Could you check a few things on this drawing? It's one solid part, dimensions in mm from its lowest x, y, z. A direction names the side the tool comes from. Give positions to 0.01 mm unless a question says otherwise; leave off trailing zeros. Write each loop counter-clockwise with the first axis right and the second up, starting at its lowest first coordinate (ties: lowest second). Pieces come first, ordered by that corner, then holes. Notation, with made-up numbers: (71, -13) -> (115, -13) arc R38 cw to (115, 26) -> close; hole circle Ø2 at (62, 39). An arc over 180 degrees is marked (long way). Use CSV: the item, a comma, the result in double quotes. Start each with the question number.
(1) I need wall thicknesses on L1, parallel to Y at x = 14, z = 4 (1 decimal); L2, parallel to Z at x = 11.75, y = 17.5 (1 decimal); L3, parallel to Y at x = 10.5, z = 8 (1 decimal). Which ranges of each line are inside material? Lowest first, please. Write a range as [from, to].
(2) Suppose I cut it at B-B on z = 4.25. List the corners of the cut face in (x, y) for me (1 decimal).
(3) Suppose I cut it at A-A on x = 3.25. List the corners of the cut face in (y, z) for me (1 decimal), plus the area to 3 significant figures.
(4) Which directions (+Z, -Z, +X, -X, +Y, -Y) give clear straight access to the entire face, cutting with the end or side of a thin tool? Please do the marked faces 1, 2 and 3.
(5) For pin 1 Ø3 at (x, y) = (3.5, 19) entering from +Z; pin 2 Ø4 at (y, z) = (5.5, 2.5) entering from +X; pin 3 Ø1.5 at (x, z) = (1.5, 6) entering from -Y, each with a flat end and sliding along its axis, tell me the tip position at first contact or that it passes through.
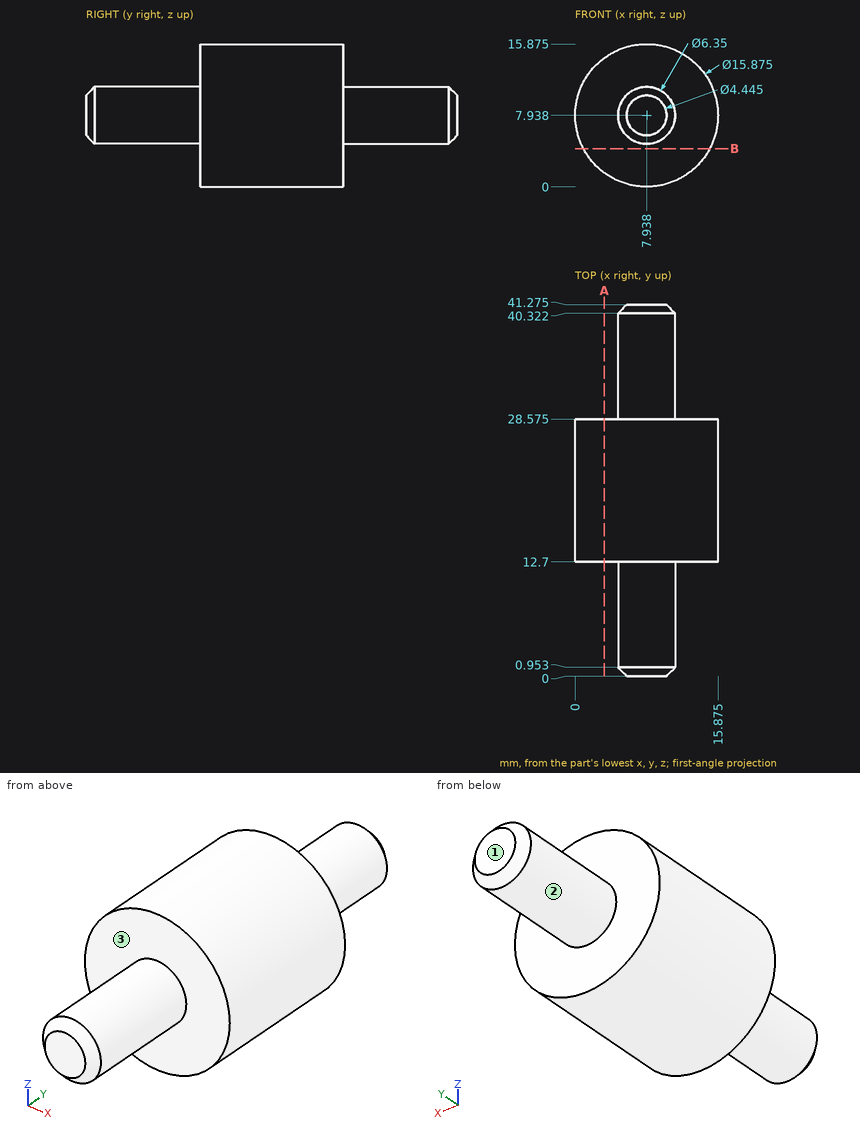
Geometry says:
1,L1,"[12.7, 28.6]"
1,L2,"[1, 14.9]"
1,L3,"[0.3, 40.9]"
2,outline,"(0.9, 12.7) -> (15, 12.7) -> (15, 28.6) -> (0.9, 28.6) -> close"
3,outline,"(12.7, 1.5) -> (28.6, 1.5) -> (28.6, 14.3) -> (12.7, 14.3) -> close"
3,area,"203 mm²"
4,face 1,"+Z, -Z, +X, -X, +Y"
4,face 2,"+Y"
4,face 3,"-Y"
5,pin 1,"z = 15.31"
5,pin 2,"through"
5,pin 3,"y = 12.7"
